Autodesk Inventor part; units mm, degrees
ref_plane "YZ Plane" through (0, 0, 0) normal (1, 0, 0) x (0, 1, 0)
ref_plane "XZ Plane" through (0, 0, 0) normal (0, 1, 0) x (-1, 0, 0)
ref_plane "XY Plane" through (0, 0, 0) normal (0, 0, 1) x (1, 0, 0)
sketch "Sketch1" plane through (0, 0, 0) normal (0, 1, 0) x (-1, 0, 0)
  line L0 (17.5, -17.5) -> (-17.5, -17.5) construction
  line L1 (-17.5, -17.5) -> (-17.5, 17.5) construction
  line L2 (-17.5, 17.5) -> (17.5, 17.5) construction
  line L3 (17.5, 17.5) -> (17.5, -17.5) construction
  line L4 (17.5, 17.5) -> (2.6797, 17.5)
  line L5 (2.6797, 17.5) -> (-17.5, -10.9168)
  line L6 (-17.5, -10.9168) -> (-17.5, -17.5)
  line L7 (-17.5, -17.5) -> (17.5, -17.5)
  line L8 (17.5, -17.5) -> (17.5, 17.5)
  point P0 (0, 0)
  dimension "d0" = 35
  dimension "d1" = 35
  dimension "d2" = 17.5
  dimension "d3" = 17.5
extrude "Extrusion1" add sketch "Sketch1" along normal blind 1
sketch "Sketch2" plane through (-17.5, 0, -17.5) normal (-1, 0, 0) x (0, 0, 1)
  line L0 (35, 35) -> (0, 35) construction
  line L1 (0, 35) -> (0, 0) construction
  line L2 (0, 0) -> (35, 0) construction
  line L3 (35, 0) -> (35, 35)
  line L4 (35, 0) -> (35, 6.1852)
  line L5 (35, 6.1852) -> (3.9768, 35)
  line L6 (3.9768, 35) -> (0, 35)
  line L7 (0, 35) -> (0, 0)
  line L8 (0, 0) -> (35, 0)
  point P0 (17.5, 0)
  dimension "d6" = 35
  dimension "d7" = 35
  dimension "d8" = 35
extrude "Extrusion2" add sketch "Sketch2" along normal blind 1
sketch "Sketch3" plane through (17.5, 0, -17.5) normal (0, 0, -1) x (-1, 0, 0)
  line L0 (35, 0) -> (35, 35)
  line L1 (35, 35) -> (29.2734, 35)
  line L2 (29.2734, 35) -> (0, 3.6651)
  line L3 (0, 3.6651) -> (0, 0)
  line L4 (0, 0) -> (35, 0)
  point P0 (17.5, 0)
  dimension "d11" = 35
  dimension "d12" = 35
extrude "Extrusion3" add sketch "Sketch3" against normal blind 1
properties part number "corner_protectipt"
Can you work these out from the model? Positions are in its coordinate system, mm. A direction names the side the tool comes from. Give positions to 0.01 mm unless a question says otherwise; leave off trailing zeros. Order: outer loops, then holes, each group sorted by start corner. A loop starts at its lowest first (then second) coordinate and runs counter-clockwise, first axis right, second up. Notation, with made-up numbers: M 45,77.25 L 79,77.25 A15 ccw 79,90.25 Z; hole C 37,27 d2. An arc over 180 degrees is marked long. Use a Markdown table: item, result. Add a question column.
Item 1: For faces 4 (the flat face through (-4, 14, -16.5)), 5 (the flat face through (-18.5, 14, -4)), which set-ups out of +Z, -Z, +X, -X, +Y, -Y let a thin tool reach every point of the face, with its end or its side?
Item 2: Suppose I cut it at B-B (y = 25). List the corners of the cut face in (x, z) for me, then the cut area to 3 significant figures.
Item 3: Will this pin go through, and if not, where does the flat tip stop? pin 1 (1.5 mm diameter, centred on x = 12, z = -11, fed in from +Y).
Item 4: We'd pull the mould along Y, two halves only. Please class faces 1 (the flat face through (-4, 1, -3)), 2 (the flat face through (-4, 0, -4)), 3 (the flat face through (-17.5, 14, -4)): +Y half, -Y half, draft (parallel to the pull), parting line (faces both ways), or undercut.
Item 5: If I drill on L1, parallel to X at y = 16, z = 2; L2, parallel to Y at x = 2.5, z = 1; L3, parallel to Z at x = -2.5, y = 12, over which ranges is the centre line in solid material (lowest first)? Write a range as [from, to].
Item 6: Suppose I cut it at A-A (z = 5). List the corners of the cut face in (x, y) for me.
Answer sheet:
| question | item | result |
|---|---|---|
| 1 | face 4 | +Z, +X, +Y |
| 1 | face 5 | +Z, -Z, -X, +Y, -Y |
| 2 | outline | M -18.5,-17.5 L -2.43,-17.5 L -2.43,-16.5 L -17.5,-16.5 L -17.5,-2.76 L -18.5,-2.76 Z |
| 2 | area | 29.8 mm² |
| 3 | pin 1 | stops at y = 1 |
| 4 | face 1 | +Y half |
| 4 | face 2 | -Y half |
| 4 | face 3 | draft |
| 5 | L1 | x = [-18.5, -17.5] |
| 5 | L2 | y = [0, 1] |
| 5 | L3 | z = [-17.5, -16.5] |
| 6 | outline | M -18.5,0 L 6.2,0 L 6.2,1 L -17.5,1 L -17.5,17.8 L -18.5,17.8 Z |
